Drawing for the job (mm, zero at the part's lowest x, y, z). Give positions to 0.01 mm unless a question says otherwise; leave off trailing zeros. Loops run counter-clockwise (first coordinate to the right, second up) from the corner with the lowest first, then second, coordinate; pieces in that order, holes last.
1) Band-saw the part on A-A on x = 13.5. List the corners of the cut face in (y, z).
2) Wall check: line 1 (Y direction, x = 10, z = 2.5); line 2 (Y direction, x = 14.5, z = 1.4) (3 decimals); line 3 (Z direction, x = 11.5, y = 3). Give the ranges that are in metal, low to high.
3) Band-saw the part on B-B on z = 2.5. List the corners of the cut face in (x, y), then the cut area to 3 significant figures.
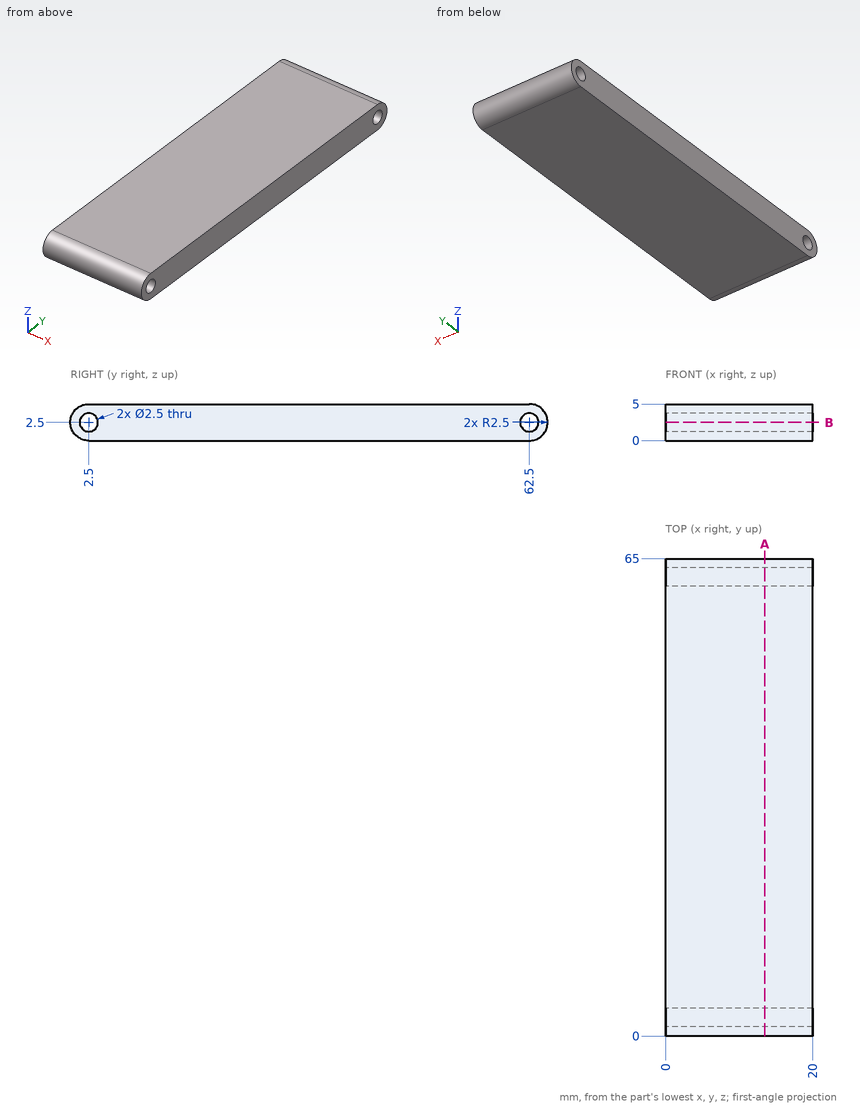
Findings below:
1. outline: (2.5, 0) - (62.5, 0) arc R2.5 ccw to (62.5, 5) - (2.5, 5) arc R2.5 ccw to start; hole circle Ø2.5 at (2.5, 2.5); hole circle Ø2.5 at (62.5, 2.5)
2. line 1: y = 0 to 1.25, 3.75 to 61.25, 63.75 to 65
2. line 2: y = 0.255 to 1.906, 3.094 to 61.906, 63.094 to 64.745
2. line 3: z = 0 to 1.35, 3.65 to 5
3. outline: (0, 0) - (20, 0) - (20, 1.25) - (0, 1.25) - close; (0, 3.75) - (20, 3.75) - (20, 61.25) - (0, 61.25) - close; (0, 63.75) - (20, 63.75) - (20, 65) - (0, 65) - close
3. area: 1,200 mm2
